The model under review builds one solid part; all positions refer to its coordinate system, in mm. A direction names the side the tool comes from. Coordinates: 2 decimals unless noted, no trailing zeros. Write each loop counter-clockwise with the first axis right and the second up, starting at its lowest first coordinate (ties: lowest second). Pieces come first, ordered by that corner, then holes. Notation, with made-up numbers: (69.5, 52) - (114.5, 52) arc R8 ccw to (114.5, 62) - close; hole circle Ø3 at (-21, 1.25). An arc over 180 degrees is marked (long way). Use one line per item in the form item = value. Start each with the question number.
```python
from build123d import *

# Parameters (mm, degrees)
BOSS_EXTRUDE2_DEPTH = 12.7
CUT_EXTRUDE3_DEPTH  = 12.7
SKETCH7_R           = 3.175
CUT_EXTRUDE5_DEPTH  = 2.54


with BuildPart() as part:
    # Sketch5 → Boss-Extrude2 (new body)
    with BuildSketch(Plane.XY):
        Polygon((17.316446729, -7.015021533), (17.542582687, 5.684978467), (8.722228835, 14.825136857), (-3.977771165, 15.051272815), (-13.117929555, 6.230918963), (-13.344065513, -6.469081037), (-4.523711662, -15.609239427), (8.176288338, -15.835375385), align=None)
    extrude(amount=BOSS_EXTRUDE2_DEPTH)

    # Sketch6 → Cut-Extrude3 (cut)
    with BuildSketch(Plane(origin=(17.435827988, -0.310462021, 0), x_dir=(0, 0, -1), z_dir=(0.9998415112072249, -0.017803158900963578, 0))):
        with BuildLine():
            ThreePointArc((-8.14590888, 1.441577842), (-8.89, -0.354615715), (-8.14590888, -2.150809272))
            Line((-8.14590888, -2.150809272), (-6.35, -0.354615715))
            Line((-6.35, -0.354615715), (-8.14590888, 1.441577842))
        make_face()
        with BuildLine():
            Line((-6.35, -0.354615715), (-8.14590888, -2.150809272))
            ThreePointArc((-8.14590888, -2.150809272), (-6.35, -2.894615715), (-4.55409112, -2.150809272))
            Line((-4.55409112, -2.150809272), (-6.35, -0.354615715))
        make_face()
        with BuildLine():
            Line((-8.14590888, 1.441577842), (-6.35, -0.354615715))
            Line((-6.35, -0.354615715), (-4.55409112, 1.441577842))
            ThreePointArc((-4.55409112, 1.441577842), (-6.35, 2.185384285), (-8.14590888, 1.441577842))
        make_face()
        with BuildLine():
            Line((-4.55409112, 1.441577842), (-6.35, -0.354615715))
            Line((-6.35, -0.354615715), (-4.55409112, -2.150809272))
            ThreePointArc((-4.55409112, -2.150809272), (-4.003384506, -1.326724619), (-3.81, -0.354615715))
            ThreePointArc((-3.81, -0.354615715), (-4.003384506, 0.617493189), (-4.55409112, 1.441577842))
        make_face()
    extrude(amount=-CUT_EXTRUDE3_DEPTH, mode=Mode.SUBTRACT)

    # Sketch7 → Cut-Extrude5 (cut)
    with BuildSketch(Plane(origin=(0, 0, 0), x_dir=(-1, 0, 0), z_dir=(0, 0, -1))):
        with Locations((-2.099258587, -0.392051285)):
            Circle(SKETCH7_R)
    extrude(amount=-CUT_EXTRUDE5_DEPTH, mode=Mode.SUBTRACT)


solid = part.part
```
1. Take a section at D-D (y = 13). State the section outline as (x, z) points, plus the area to 3 significant figures.
2. For P1, Ø4, axis at x = 8.5, z = 8.5, coming from the +Y side; P2, Ø3, axis at y = -8, z = 10.5, coming from the +X side; P3, Ø1.5, axis at y = 3.5, z = 6.5, coming from the +X side; P4, Ø5, axis at x = -7, y = -4, coming from the -Z side, all flat-tipped, find the tip position at first contact; note any pin that passes through.
3. Take a section at C-C (z = 10). State the section outline as (x, y) points.
4. For L1, parallel to Y at x = 11, z = 4.5; L2, parallel to Y at x = 9.5, z = 5.25; L3, parallel to X at y = 13, z = 8.5, list the stretches that pass through material, from the lowest coordinate up.
5. Take a section at B-B (x = 3.5). State the section outline as (y, z) points.
6. For faces 1 (the flat face through (2, 0, 2.54)), 2 (the flat face through (2, 0, 12.7)), list the 3-axis set-ups (+Z, -Z, +X, -X, +Y, -Y) from which the entire face can be reached by the end or side of a thin tool; tool diameter is ignored.
7. The part is to be moulded in two halves that separate along X. For faces 3 (the cylindrical face through (-0.93, 0.56, 1.25)), 4 (the flat face through (12.68, -11.49, 6.26)), 5 (the flat face through (-2, 0, 0)), say which applies: released by +X, released by -X, zero draft, split by the parting line, or undercut.
8. Take a section at A-A (z = 2). State the section outline as (x, y) points (3 decimals), plus the area to 3 significant figures.
Returned:
q1.outline = (-6.1, 0) - (10.48, 0) - (10.48, 12.7) - (-6.1, 12.7) - close
q1.area = 211 mm²
q2.P1 = 14.86
q2.P2 = 17.33
q2.P3 = 17.52
q2.P4 = 0
q3.outline = (-13.34, -6.47) - (-4.52, -15.61) - (8.18, -15.84) - (17.32, -7.02) - (17.54, 5.68) - (8.72, 14.83) - (-3.98, 15.05) - (-13.12, 6.23) - close
q4.L1 = -13.11 to -2.29, 1.19 to 12.46
q4.L2 = -14.56 to -2.81, 1.77 to 14.02
q4.L3 = -6.1 to 10.48
q5.outline = (-15.75, 0) - (-3.24, 0) - (-3.24, 2.54) - (2.46, 2.54) - (2.46, 0) - (14.92, 0) - (14.92, 12.7) - (-15.75, 12.7) - close
q6.face_1 = -Z
q6.face_2 = +Z, +X, -X, +Y, -Y
q7.face_3 = undercut
q7.face_4 = released by +X
q7.face_5 = zero draft
q8.outline = (-13.344, -6.469) - (-4.524, -15.609) - (8.176, -15.835) - (17.316, -7.015) - (17.543, 5.685) - (8.722, 14.825) - (-3.978, 15.051) - (-13.118, 6.231) - close; hole circle Ø6.35 at (2.099, -0.392)
q8.area = 747 mm²
